from build123d import *

# Parameters (mm, degrees)
BASPROSKE_W     = 50.8
BASPROSKE_H     = 63.5
TOOTHCUT_DEPTH  = 104.175287739
TEETHCUTS_COUNT = 18
BORSKE_R        = 12.7
BORE_DEPTH      = 50.8000508


with BuildPart() as part:
    # BasProSke → Base-Revolve (revolve)
    with BuildSketch(Plane(origin=(0, 0, 0), x_dir=(1, 0, 0), z_dir=(0, 1, 0)), mode=Mode.PRIVATE) as base_revolve_sk:
        with Locations((25.4, 31.75)):
            Rectangle(BASPROSKE_W, BASPROSKE_H)
    revolve(base_revolve_sk.sketch.rotate(Axis((-10, 0, 0), (1, 0, 0)), 180), axis=Axis((-10, 0, 0), (1, 0, 0)))

    # TooCutSke → ToothCut (cut, through all)
    with BuildSketch(Plane(origin=(0, 0, 0), x_dir=(0, 0, -1), z_dir=(1, 0, 0))):
        with BuildLine():
            ThreePointArc((3.223886101, 49.105516152), (0, 49.21123), (-3.223886101, 49.105516152))
            ThreePointArc((-3.223886101, 49.105516152), (-5.190584502, 56.49010796), (-9.481297068, 62.813863526))
            ThreePointArc((-9.481297068, 62.813863526), (0, 63.5254), (9.481297068, 62.813863526))
            ThreePointArc((9.481297068, 62.813863526), (5.190584502, 56.49010796), (3.223886101, 49.105516152))
        make_face()
    toothcut = extrude(amount=TOOTHCUT_DEPTH, mode=Mode.SUBTRACT)

    # TeethCuts: ToothCut ×18 about axis
    teethcuts_axis = Axis((0, 0, 0), (1, 0, 0))
    for i in range(1, TEETHCUTS_COUNT):
        add(toothcut.rotate(teethcuts_axis, i * 360 / TEETHCUTS_COUNT), mode=Mode.SUBTRACT)

    # BorSke → Bore (cut, symmetric)
    with BuildSketch(Plane(origin=(0, 0, 0), x_dir=(0, 0, -1), z_dir=(1, 0, 0))):
        with Locations(Location((0, 0, 0), (0, 0, 180))):
            Circle(BORSKE_R)
    extrude(amount=BORE_DEPTH, both=True, mode=Mode.SUBTRACT)


solid = part.part
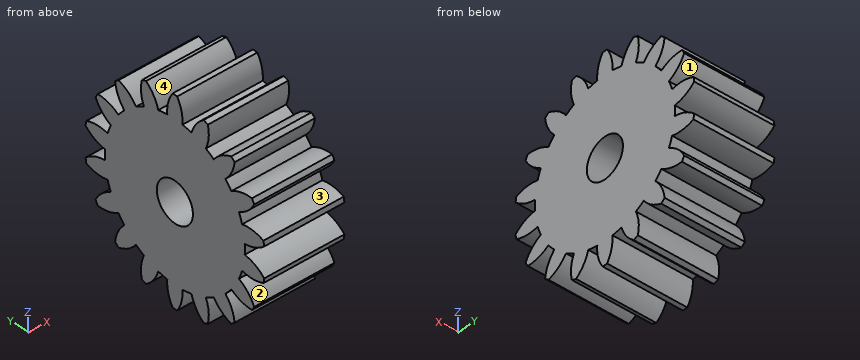
Model file for the job. Use its own axes, mm. Face numbers are marked on the shaded views. A direction names the side the tool comes from. Give positions to 0.01 mm unless a question says otherwise; leave off trailing zeros. Loops run counter-clockwise (first coordinate to the right, second up) from the corner with the lowest first, then second, coordinate; pieces in that order, holes last.
1) Saw through at C-C (y = 15.5). Write the cut outline in (x, z), plus the area to 3 significant figures.
2) Flat gauge pins, fed straight in: pin 1 Ø23 at (y, z) = (0, 0) entering from +X; pin 2 Ø3 at (x, z) = (11, 44.5) entering from +Y; pin 3 Ø10 at (x, z) = (21.5, -36.5) entering from -Y; pin 4 Ø1.5 at (x, y) = (43.5, -7) entering from -Z. Where does each tip first touch, or does it go through?
3) Saw through at B-B (y = 0). Write the cut outline in (x, z), plus the area to 3 significant figures.
4) Saw through at A-A (z = 0). Write the cut outline in (x, y).
5) Tool access for the marked faces 1, 2, 3 and 4: list every direction of +Z, -Z, +X, -X, +Y, -Y with a clear straight run to the whole face (end or side of a thin tool).
6) Wall check: line 1 (Y direction, x = 14, z = 0); line 2 (Y direction, x = 24, z = 52.5); line 3 (Z direction, x = 31, y = -38.5). Give the ranges that are in metal, low to high.
Answer block:
1. outline: (0, -55.53) - (50.8, -55.53) - (50.8, 55.53) - (0, 55.53) - close
1. area: 5,640 mm2
2. pin 1: passes through
2. pin 2: stops at y = 41.78
2. pin 3: stops at y = -55.14
2. pin 4: stops at z = -48.81
3. outline: (0, -63.5) - (50.8, -63.5) - (50.8, -12.7) - (0, -12.7) - close; (0, 12.7) - (50.8, 12.7) - (50.8, 63.5) - (0, 63.5) - close
3. area: 5,160 mm2
4. outline: (0, -49.21) - (50.8, -49.21) - (50.8, -12.7) - (0, -12.7) - close; (0, 12.7) - (50.8, 12.7) - (50.8, 49.21) - (0, 49.21) - close
5. face 1: +X, -X, +Y
5. face 2: +X, -X, -Y
5. face 3: +X, -X
5. face 4: +Z, +X, -X
6. line 1: y = -49.21 to -12.7, 12.7 to 49.21
6. line 2: y = -23.82 to -13.57, -5.37 to 5.37, 13.57 to 23.82
6. line 3: z = -49.3 to -37.71, -30.65 to 30.65, 37.71 to 49.3
